Geometry check sheet. Reference: drawing and pictorial views, mm from the part's lowest x, y, z. Round coordinates to 2 decimals unless told otherwise and drop trailing zeros. Write each loop counter-clockwise with the first axis right and the second up, starting at its lowest first coordinate (ties: lowest second). Pieces come first, ordered by that corner, then holes. Notation, with made-up numbers: M 10,34 L 20,34 A6 ccw 20,42 Z; hole C 12,-40 d10. An arc over 180 degrees is marked long. One line per item, written item: value. Start each with the question number.
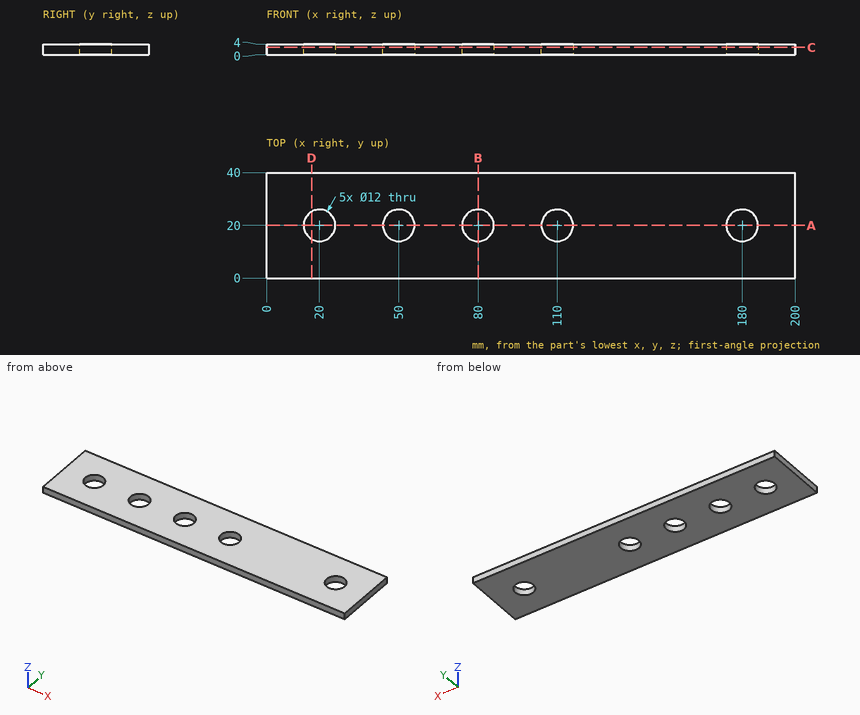
1) Gauge pin test, flat end, axial feed: pin 1 Ø9.5 at (x, y) = (180, 20) entering from +Z. Record the tip position at first contact, or that the pin passes through.
2) Thickness scan on line 1 (Y direction, x = 80, z = 1.35); line 2 (X direction, y = 21, z = 1.7); line 3 (X direction, y = 18, z = 1.5). Record the ranges inside material, lowest first.
3) Cross-section at D-D (x = 17). Record the boundary of the cut face in (y, z).
4) Cross-section at A-A (y = 20). Record the boundary of the cut face in (x, z), then the cut area to 3 significant figures.
5) Cross-section at B-B (x = 80). Record the boundary of the cut face in (y, z), then the cut area to 3 significant figures.
6) Cross-section at C-C (z = 2.7). Record the boundary of the cut face in (x, y).
Results below:
1. pin 1: passes through
2. line 1: y = 0 to 14, 26 to 40
2. line 2: x = 0 to 14.08, 25.92 to 44.08, 55.92 to 74.08, 85.92 to 104.08, 115.92 to 174.08, 185.92 to 200
2. line 3: x = 0 to 14.34, 25.66 to 44.34, 55.66 to 74.34, 85.66 to 104.34, 115.66 to 174.34, 185.66 to 200
3. outline: M 0,0 L 14.8,0 L 14.8,4 L 0,4 Z; M 25.2,0 L 40,0 L 40,4 L 25.2,4 Z
4. outline: M 0,0 L 14,0 L 14,4 L 0,4 Z; M 26,0 L 44,0 L 44,4 L 26,4 Z; M 56,0 L 74,0 L 74,4 L 56,4 Z; M 86,0 L 104,0 L 104,4 L 86,4 Z; M 116,0 L 174,0 L 174,4 L 116,4 Z; M 186,0 L 200,0 L 200,4 L 186,4 Z
4. area: 560 mm²
5. outline: M 0,0 L 14,0 L 14,4 L 0,4 Z; M 26,0 L 40,0 L 40,4 L 26,4 Z
5. area: 112 mm²
6. outline: M 0,0 L 200,0 L 200,40 L 0,40 Z; hole C 20,20 d12; hole C 50,20 d12; hole C 80,20 d12; hole C 110,20 d12; hole C 180,20 d12
